Read the model definition and answer for the solid it produces. Units are mm, in the model's axes. Round coordinates to 2 decimals unless told otherwise and drop trailing zeros. Order: outer loops, then holes, each group sorted by start corner. A loop starts at its lowest first (then second) coordinate and runs counter-clockwise, first axis right, second up. Notation, with made-up numbers: M 64.5,23 L 84.5,23 A11 ccw 84.5,41 Z; hole C -28.75,-20.5 d1. An arc over 180 degrees is marked long. Answer as CSV lines item,"result".
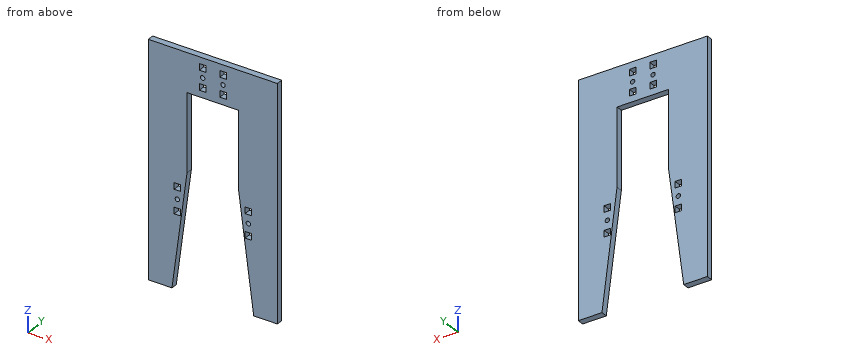
```python
from build123d import *

# Parameters (mm, degrees)
BOTTOM_PLATE_R      = 2.159
BOTTOM_PLATE_R_2    = 2.794
BOTTOM_PLATE_W      = 25.4
BOTTOM_PLATE_H      = 101.6
BOTTOM_PLATE_W_2    = 6.35
BOTTOM_PLATE_H_2    = 6.35
BOSS_EXTRUDE1_DEPTH = 6.35
SKETCH1_W           = 508
SKETCH1_H           = 508
SKETCH1_W_2         = 127
SKETCH1_H_2         = 228.6
CUT_EXTRUDE1_DEPTH  = 25.4


with BuildPart() as part:
    # Bottom Plate → Boss-Extrude1 (new body)
    # profile 1 of 3: a face of its own
    with BuildSketch(Plane(origin=(0, 0, 0), x_dir=(1, 0, 0), z_dir=(0, 1, 0))):
        with BuildLine():
            Line((25.4, 0), (47.625, 171.302946195))
            ThreePointArc((47.625, 171.302946195), (0, -177.8), (-47.625, 171.302946195))
            Line((-47.625, 171.302946195), (-25.4, 0))
            Line((-25.4, 0), (-25.4, -76.2))
            Line((-25.4, -76.2), (25.4, -76.2))
            Line((25.4, -76.2), (25.4, 0))
        make_face()
        with Locations((128.515324336, 72.009)):
            Circle(BOTTOM_PLATE_R, mode=Mode.SUBTRACT)
        with Locations((128.515324336, -72.009)):
            Circle(BOTTOM_PLATE_R, mode=Mode.SUBTRACT)
        with Locations((54.082553747, 147.04477289)):
            Circle(BOTTOM_PLATE_R, mode=Mode.SUBTRACT)
        with Locations(Location((34.925, 28.321, 0), (0, 0, 270))):
            Circle(BOTTOM_PLATE_R, mode=Mode.SUBTRACT)
        with Locations(Location((-10.033, -95.25, 0), (0, 0, 270))):
            Circle(BOTTOM_PLATE_R, mode=Mode.SUBTRACT)
        with Locations((27.813, -127)):
            Circle(BOTTOM_PLATE_R_2, mode=Mode.SUBTRACT)
        with Locations((-27.813, -127)):
            Circle(BOTTOM_PLATE_R_2, mode=Mode.SUBTRACT)
        with Locations(Location((10.033, -95.25, 0), (0, 0, 90))):
            Circle(BOTTOM_PLATE_R, mode=Mode.SUBTRACT)
        with Locations(Location((-34.925, 28.321, 0), (0, 0, 90))):
            Circle(BOTTOM_PLATE_R, mode=Mode.SUBTRACT)
        with Locations((-128.515324336, -72.009)):
            Circle(BOTTOM_PLATE_R, mode=Mode.SUBTRACT)
        with Locations((-128.515324336, 72.009)):
            Circle(BOTTOM_PLATE_R, mode=Mode.SUBTRACT)
        with Locations((-54.082553747, 147.04477289)):
            Circle(BOTTOM_PLATE_R, mode=Mode.SUBTRACT)
        with Locations((144.390324336, 0)):
            Rectangle(BOTTOM_PLATE_W, BOTTOM_PLATE_H, mode=Mode.SUBTRACT)
        with Locations((-34.925, 40.005)):
            Rectangle(BOTTOM_PLATE_W_2, BOTTOM_PLATE_H_2, mode=Mode.SUBTRACT)
        with Locations((34.925, 16.637)):
            Rectangle(BOTTOM_PLATE_W_2, BOTTOM_PLATE_H_2, mode=Mode.SUBTRACT)
        with Locations((34.925, 40.005)):
            Rectangle(BOTTOM_PLATE_W_2, BOTTOM_PLATE_H_2, mode=Mode.SUBTRACT)
        with Locations((128.515324336, -60.325)):
            Rectangle(BOTTOM_PLATE_W_2, BOTTOM_PLATE_H_2, mode=Mode.SUBTRACT)
        with Locations((128.515324336, 60.325)):
            Rectangle(BOTTOM_PLATE_W_2, BOTTOM_PLATE_H_2, mode=Mode.SUBTRACT)
        with Locations((-34.925, 16.637)):
            Rectangle(BOTTOM_PLATE_W_2, BOTTOM_PLATE_H_2, mode=Mode.SUBTRACT)
        with Locations((-10.033, -85.725)):
            Rectangle(BOTTOM_PLATE_W_2, BOTTOM_PLATE_H_2, mode=Mode.SUBTRACT)
        with Locations((-10.033, -104.775)):
            Rectangle(BOTTOM_PLATE_W_2, BOTTOM_PLATE_H_2, mode=Mode.SUBTRACT)
        with Locations((10.033, -104.775)):
            Rectangle(BOTTOM_PLATE_W_2, BOTTOM_PLATE_H_2, mode=Mode.SUBTRACT)
        with Locations((10.033, -85.725)):
            Rectangle(BOTTOM_PLATE_W_2, BOTTOM_PLATE_H_2, mode=Mode.SUBTRACT)
        with Locations((-144.390324336, 0)):
            Rectangle(BOTTOM_PLATE_W, BOTTOM_PLATE_H, mode=Mode.SUBTRACT)
        with Locations((-128.515324336, -60.325)):
            Rectangle(BOTTOM_PLATE_W_2, BOTTOM_PLATE_H_2, mode=Mode.SUBTRACT)
        with Locations((-128.515324336, 60.325)):
            Rectangle(BOTTOM_PLATE_W_2, BOTTOM_PLATE_H_2, mode=Mode.SUBTRACT)
    # profile 2 of 3: a face of its own
    with BuildSketch(Plane(origin=(0, 0, 0), x_dir=(1, 0, 0), z_dir=(0, 1, 0))):
        Polygon((52.518937038, 159.669886307), (58.816158581, 158.852879058), (59.63316583, 165.1501006), (53.335944287, 165.967107849), align=None)
    # profile 3 of 3: a face of its own
    with BuildSketch(Plane(origin=(0, 0, 0), x_dir=(1, 0, 0), z_dir=(0, 1, 0))):
        Polygon((-58.816158581, 158.852879058), (-59.63316583, 165.1501006), (-53.335944287, 165.967107849), (-52.518937038, 159.669886307), align=None)
    extrude(amount=-BOSS_EXTRUDE1_DEPTH)

    # Sketch1 → Cut-Extrude1 (cut)
    with BuildSketch(Plane(origin=(0, 0, 0), x_dir=(1, 0, 0), z_dir=(0, 1, 0))):
        Rectangle(SKETCH1_W, SKETCH1_H)
        Rectangle(SKETCH1_W_2, SKETCH1_H_2, mode=Mode.SUBTRACT)
    extrude(amount=-CUT_EXTRUDE1_DEPTH, mode=Mode.SUBTRACT)


solid = part.part
```
Item 1: Flat-ended cylindrical pins translate along their axes: pin 1 (2 mm diameter, centred on x = 35, z = 86.5, fed in from +Y); pin 2 (2 mm diameter, centred on x = 13, y = -4, fed in from -Z). Find the tip coordinate at first contact, or state that the pin passes through.
Ans:
pin 1,"y = 0"
pin 2,"z = 76.2"
Item 2: A cutting plane is placed at D-D, the plane x = -0.5. Determine the outline of the cut face in (y, z), and give its area (3 significant figures).
Ans:
outline,"M -6.35,76.2 L 0,76.2 L 0,114.3 L -6.35,114.3 Z"
area,"242 mm2"
Item 3: A cutting plane is placed at A-A, the plane z = 95.25. Determine the outline of the cut face in (x, y).
Ans:
outline,"M -63.5,-6.35 L -12.19,-6.35 L -12.19,0 L -63.5,0 Z; M -7.87,-6.35 L 7.87,-6.35 L 7.87,0 L -7.87,0 Z; M 12.19,-6.35 L 63.5,-6.35 L 63.5,0 L 12.19,0 Z"
Item 4: A cutting plane is placed at C-C, the plane z = 26. Determine the outline of the cut face in (x, y).
Ans:
outline,"M -63.5,-6.35 L -25.4,-6.35 L -25.4,0 L -63.5,0 Z; M 25.4,-6.35 L 63.5,-6.35 L 63.5,0 L 25.4,0 Z"
Item 5: Find the intervals of material crossed by probe 1 along X at (y, z) = (-3, 95.25); probe 2 along Z at (x, y) = (12.5, -5.25); probe 3 along X at (y, z) = (-1.75, 84), in increasing order. Write a range as [from, to].
Ans:
probe 1,"[-63.5, -12.19], [-7.87, 7.87], [12.19, 63.5]"
probe 2,"[76.2, 82.55], [88.9, 101.6], [107.95, 114.3]"
probe 3,"[-63.5, -13.21], [-6.86, 6.86], [13.21, 63.5]"
Item 6: A cutting plane is placed at B-B, the plane z = -23. Determine the outline of the cut face in (x, y), and give its area (3 significant figures).
Ans:
outline,"M -63.5,-6.35 L -28.38,-6.35 L -28.38,0 L -63.5,0 Z; M 28.38,-6.35 L 63.5,-6.35 L 63.5,0 L 28.38,0 Z"
area,"446 mm2"
